from build123d import *

# Parameters (mm, degrees)
SKETCH1_W           = 82.539998569
SKETCH1_H           = 65.04
BOSS_EXTRUDE1_DEPTH = 43.18
SHELL1_T            = 2.54
SKETCH2_R           = 1.085
CUT_EXTRUDE1_DEPTH  = 124.952130409
FILLET1_R           = 6.20014
FILLET2_R           = 1
SKETCH6_W           = 35.56
SKETCH6_H           = 50.8
CUT_EXTRUDE2_DEPTH  = 124.028758627
SKETCH3_R           = 2.125
BOSS_EXTRUDE2_DEPTH = 9.39038
CUT_EXTRUDE3_DEPTH  = 2.54
SKETCH8_W           = 1.27
SKETCH8_H           = 33.02
CUT_EXTRUDE4_DEPTH  = 2.54
SKETCH10_W          = 87.619998569
SKETCH10_H          = 10.145268184
BOSS_EXTRUDE3_DEPTH = 2.54
CUT_EXTRUDE5_DEPTH  = 2.54
SKETCH11_W          = 12.7
SKETCH11_H          = 8
BOSS_EXTRUDE4_DEPTH = 12.7
SKETCH12_R          = 2.625
CUT_EXTRUDE6_DEPTH  = 127.362400741
SKETCH13_W          = 7.62
SKETCH13_H          = 12.7
BOSS_EXTRUDE5_DEPTH = 12.7
SKETCH14_R          = 2.625
CUT_EXTRUDE7_DEPTH  = 125.717897357
FILLET3_R           = 3


with BuildPart() as part:
    # Sketch1 → Boss-Extrude1 (new body)
    with BuildSketch(Plane.XY):
        with Locations((47.599999189, 40.75)):
            Rectangle(SKETCH1_W, SKETCH1_H)
    extrude(amount=BOSS_EXTRUDE1_DEPTH)

    # Shell1
    shell1_openings = [part.faces().sort_by_distance(p)[0] for p in [
        (47.599999189, 73.27, 21.59),
        (47.599999189, 40.75, 0),
    ]]
    offset(amount=SHELL1_T, openings=shell1_openings, kind=Kind.INTERSECTION)

    # Sketch2 → Cut-Extrude1 (cut, through all)
    with BuildSketch(Plane(origin=(97.099998474, 5.69, 0), x_dir=(0, 0, -1), z_dir=(0, 1, 0))):
        with Locations(Location((-10.166, 73.199999285, 0), (0, 0, 90))):
            Circle(SKETCH2_R)
        with Locations(Location((-10.166, 25.799999285, 0), (0, 0, 90))):
            Circle(SKETCH2_R)
        with Locations(Location((-28.266, 24.299999285, 0), (0, 0, 90))):
            Circle(SKETCH2_R)
        with Locations(Location((-28.266, 74.699999285, 0), (0, 0, 90))):
            Circle(SKETCH2_R)
        Polygon((-33.02, 71.391050497), (-8.912, 71.391050497), (-8.912, 55.244166488), (-6.912, 55.244166488), (-6.912, 43.755832082), (-8.912, 43.755832082), (-8.912, 27.608948073), (-33.02, 27.608948073), align=None)
    extrude(amount=CUT_EXTRUDE1_DEPTH, mode=Mode.SUBTRACT)

    # Fillet1
    fillet1_edges = [part.edges().sort_by_distance(p)[0] for p in [
        (25.708947978, 6.96, 33.02),
        (69.491050401, 6.96, 33.02),
        (69.491050401, 6.96, 8.912),
        (25.708947978, 6.96, 8.912),
    ]]
    fillet(fillet1_edges, radius=FILLET1_R)

    # Fillet2
    fillet2_edges = [part.edges().sort_by_distance(p)[0] for p in [
        (53.344166393, 6.96, 6.912),
        (41.855831986, 6.96, 6.912),
    ]]
    fillet(fillet2_edges, radius=FILLET2_R)
    fillet2_2_edges = [part.edges().sort_by_distance(p)[0] for p in [
        (53.344166393, 6.96, 8.912),
        (41.855831986, 6.96, 8.912),
    ]]
    fillet(fillet2_2_edges, radius=FILLET2_R - 0.0001)  # a hair under: the kernel refuses the full size

    # Sketch6 → Cut-Extrude2 (cut, through all)
    with BuildSketch(Plane.ZY.offset(-3.789999905)):
        with Locations((17.78, 47.87)):
            Rectangle(SKETCH6_W, SKETCH6_H)
    extrude(amount=-CUT_EXTRUDE2_DEPTH, mode=Mode.SUBTRACT)

    # Sketch3 → Boss-Extrude2 (add)
    # profile 1 of 4: a face of its own
    with BuildSketch(Plane(origin=(0, 0, 43.18), x_dir=(-1, 0, 0), z_dir=(0, 0, -1))):
        with BuildLine():
            Line((-86.514394884, 72), (-78.685601874, 72))
            ThreePointArc((-78.685601874, 72), (-78.109870373, 62.509871885), (-87.599998474, 63.085603617))
            Line((-87.599998474, 63.085603617), (-87.599998474, 70.914396383))
            ThreePointArc((-87.599998474, 70.914396383), (-87.090126494, 71.490128006), (-86.514394884, 72))
        make_face()
        with Locations(Location((-82.599998379, 67, 0), (0, 0, 180))):
            Circle(SKETCH3_R, mode=Mode.SUBTRACT)
    # profile 2 of 4: a face of its own
    with BuildSketch(Plane(origin=(0, 0, 43.18), x_dir=(-1, 0, 0), z_dir=(0, 0, -1))):
        with BuildLine():
            Line((-7.599999905, 70.914398454), (-7.599999905, 63.085601546))
            ThreePointArc((-7.599999905, 63.085601546), (-17.090127314, 62.509872815), (-16.514394884, 72))
            Line((-16.514394884, 72), (-8.685601874, 72))
            ThreePointArc((-8.685601874, 72), (-8.109871193, 71.490128936), (-7.599999905, 70.914398454))
        make_face()
        with Locations(Location((-12.599998379, 67, 0), (0, 0, 180))):
            Circle(SKETCH3_R, mode=Mode.SUBTRACT)
    # profile 3 of 4: a face of its own
    with BuildSketch(Plane(origin=(0, 0, 43.18), x_dir=(-1, 0, 0), z_dir=(0, 0, -1))):
        with BuildLine():
            Line((-7.599999905, 20.914398454), (-7.599999905, 13.085601546))
            ThreePointArc((-7.599999905, 13.085601546), (-18.949998379, 17), (-7.599999905, 20.914398454))
        make_face()
        with Locations(Location((-12.599998379, 17, 0), (0, 0, 180))):
            Circle(SKETCH3_R, mode=Mode.SUBTRACT)
    # profile 4 of 4: a face of its own
    with BuildSketch(Plane(origin=(0, 0, 43.18), x_dir=(-1, 0, 0), z_dir=(0, 0, -1))):
        with BuildLine():
            Line((-87.599998474, 20.914396383), (-87.599998474, 13.085603617))
            ThreePointArc((-87.599998474, 13.085603617), (-76.249998379, 17), (-87.599998474, 20.914396383))
        make_face()
        with Locations(Location((-82.599998379, 17, 0), (0, 0, 180))):
            Circle(SKETCH3_R, mode=Mode.SUBTRACT)
    extrude(amount=BOSS_EXTRUDE2_DEPTH)

    # Sketch7 → Cut-Extrude3 (cut)
    with BuildSketch(Plane(origin=(0, 0, 0), x_dir=(-1, 0, 0), z_dir=(0, 0, -1))):
        Polygon((-91.409998474, 22.47), (-90.139998474, 22.47), (-90.139998474, 6.96), (-5.059999905, 6.96), (-5.059999905, 22.47), (-3.789999905, 22.47), (-3.789999905, 5.69), (-91.409998474, 5.69), align=None)
    extrude(amount=-CUT_EXTRUDE3_DEPTH, mode=Mode.SUBTRACT)

    # Sketch8 → Cut-Extrude4 (cut)
    with BuildSketch(Plane(origin=(0, 22.47, 0), x_dir=(1, 0, 0), z_dir=(0, 1, 0))):
        with Locations((4.424999905, -19.05)):
            Rectangle(SKETCH8_W, SKETCH8_H)
        with Locations((90.774998474, -19.05)):
            Rectangle(SKETCH8_W, SKETCH8_H)
    extrude(amount=-CUT_EXTRUDE4_DEPTH, mode=Mode.SUBTRACT)

    # Sketch10 → Boss-Extrude3 (add)
    with BuildSketch(Plane(origin=(0, 73.27, 0), x_dir=(1, 0, 0), z_dir=(0, 1, 0))):
        with Locations((47.59999919, -40.647365908)):
            Rectangle(SKETCH10_W, SKETCH10_H)
    extrude(amount=BOSS_EXTRUDE3_DEPTH)

    # Sketch9 → Cut-Extrude5 (cut)
    with BuildSketch(Plane(origin=(0, 0, 35.56), x_dir=(-1, 0, 0), z_dir=(0, 0, -1))):
        Polygon((-90.139998474, 73.27), (-90.139998474, 74.54), (-5.059999905, 74.54), (-5.059999905, 73.27), (-5.059999905, 19.93), (-3.789999905, 19.93), (-3.789999905, 73.27), (-3.789999905, 75.81), (-91.409998474, 75.81), (-91.409998474, 73.27), (-91.409998474, 19.93), (-90.139998474, 19.93), align=None)
    extrude(amount=-CUT_EXTRUDE5_DEPTH, mode=Mode.SUBTRACT)

    # Sketch11 → Boss-Extrude4 (add)
    with BuildSketch(Plane.XZ.offset(-5.69)):
        with Locations((83.789998474, 6.54)):
            Rectangle(SKETCH11_W, SKETCH11_H)
        with Locations((11.409999905, 6.54)):
            Rectangle(SKETCH11_W, SKETCH11_H)
    extrude(amount=BOSS_EXTRUDE4_DEPTH)

    # Sketch12 → Cut-Extrude6 (cut, through all)
    with BuildSketch(Plane(origin=(0, 0, 2.54), x_dir=(-1, 0, 0), z_dir=(0, 0, -1))):
        with Locations((-83.789998474, -0.66)):
            Circle(SKETCH12_R)
        with Locations((-11.409999905, -0.66)):
            Circle(SKETCH12_R)
    extrude(amount=-CUT_EXTRUDE6_DEPTH, mode=Mode.SUBTRACT)

    # Sketch13 → Boss-Extrude5 (add)
    with BuildSketch(Plane.ZY.offset(-3.789999905)):
        with Locations((41.91, 69.46)):
            Rectangle(SKETCH13_W, SKETCH13_H)
    boss_extrude5 = extrude(amount=BOSS_EXTRUDE5_DEPTH)

    # Sketch14 → Cut-Extrude7 (cut, through all)
    with BuildSketch(Plane(origin=(0, 0, 38.1), x_dir=(-1, 0, 0), z_dir=(0, 0, -1))):
        with Locations(Location((2.560000095, 69.46, 0), (0, 0, 90))):
            Circle(SKETCH14_R)
    cut_extrude7 = extrude(amount=-CUT_EXTRUDE7_DEPTH, mode=Mode.SUBTRACT)

    # Mirror1: Boss-Extrude5, Cut-Extrude7 across plane
    add(boss_extrude5.mirror(Plane.ZY.offset(-47.599999189)))
    add(cut_extrude7.mirror(Plane.ZY.offset(-47.599999189)), mode=Mode.SUBTRACT)

    # Fillet3
    fillet3_edges = [part.edges().sort_by_distance(p)[0] for p in [
        (6.329999905, 73.27, 39.377365908),
        (6.329999905, 8.23, 21.59),
        (88.869998474, 8.23, 21.59),
        (88.869998474, 73.27, 39.377365908),
        (17.759999905, 5.69, 6.54),
        (17.759999905, -7.01, 6.54),
        (5.059999905, -7.01, 6.54),
        (77.439998474, 5.69, 6.54),
        (90.139998474, -7.01, 6.54),
        (77.439998474, -7.01, 6.54),
        (3.789999905, 63.11, 41.91),
        (-8.910000095, 63.11, 41.91),
        (-8.910000095, 75.81, 41.91),
        (104.109998474, 75.81, 41.91),
        (104.109998474, 63.11, 41.91),
        (91.409998474, 63.11, 41.91),
        (91.409998474, 5.69, 24.13),
        (3.789999905, 5.69, 24.13),
    ]]
    fillet(fillet3_edges, radius=FILLET3_R)


solid = part.part
Here's how the part is built. I have some questions about the finished solid (model axes, mm). A direction names the side the tool comes from. Give positions to 0.01 mm unless a question says otherwise; leave off trailing zeros. Order: outer loops, then holes, each group sorted by start corner. A loop starts at its lowest first (then second) coordinate and runs counter-clockwise, first axis right, second up. Notation, with made-up numbers: (56, -2.5) -> (91, -2.5) arc R20 cw to (91, 1.5) -> close; hole circle Ø3 at (33.25, 0.25). An arc over 180 degrees is marked (long way). Use a Markdown table: item, result. Add a question column.
Item 1: Imagine slicing it at D-D on y = 45.5. Please give me the cut outline in (x, z), plus the area to 3 significant figures.
Item 2: Imagine slicing it at C-C on z = 20. Please give me the cut outline in (x, y), plus the area to 3 significant figures.
Item 3: For faces 1 (the face through (7.23, 9.09, 21.89)), 2 (the face through (67.63, 6.98, 31.25)), 3 (the face through (98, 63.11, 42)), which set-ups out of +Z, -Z, +X, -X, +Y, -Y let a thin tool reach every point of the face, with its end or its side?
Item 4: Imagine slicing it at A-A on x = -2.56. Please give me the cut outline in (y, z) (3 decimals).
Item 5: If we mould it in two halves opening along X, with no side actions, what happens to faces 4 (the face through (8.906, 0.128, 6.484)), 5 (the face through (103.21, 63.97, 41.96)), 6 (the face through (78.3, -6.11, 6.6)), 7 (the face through (-8.01, 74.95, 41.96))? For each: pulls with the +X half, pulls with the -X half, needs draft (parallel to the pull), parting line crosses it, or undercut.
Item 6: I need wall thicknesses on line 1 (X direction, y = -1, z = 3); line 2 (Z direction, x = 72.8, y = 7.3); line 3 (X direction, y = 12.5, z = 31.5). Which ranges of each line are inside material? Lowest first, please.
Item 7: Will these pins go through, and if not, where does the flat tip stop? pin 1 (5 mm diameter, centred on x = 71, y = 43.5, fed in from -Z); pin 2 (12.5 mm diameter, centred on x = 13.5, y = 19, fed in from -Z); pin 3 (2 mm diameter, centred on y = 7, z = 21.5, fed in from +X); pin 4 (13 mm diameter, centred on x = 34, z = 16, fed in from +Y).
Item 8: Imagine slicing it at B-B on y = -0.66. Please give me the cut outline in (x, z) (3 decimals), plus the area to 3 significant figures.
Data:
| question | item | result |
|---|---|---|
| 1 | outline | (3.79, 38.1) -> (5.06, 38.1) -> (5.06, 35.56) -> (6.33, 35.56) -> (6.33, 43.18) -> (88.87, 43.18) -> (88.87, 35.56) -> (90.14, 35.56) -> (90.14, 38.1) -> (91.41, 38.1) -> (91.41, 45.72) -> (3.79, 45.72) -> close |
| 1 | area | 255 mm² |
| 2 | outline | (3.79, 8.69) arc R3 ccw to (6.79, 5.69) -> (25.71, 5.69) -> (25.71, 8.23) -> (9.33, 8.23) arc R3 cw to (6.33, 11.23) -> (6.33, 22.47) -> (5.06, 22.47) -> (5.06, 19.93) -> (3.79, 19.93) -> close; (69.49, 5.69) -> (88.41, 5.69) arc R3 ccw to (91.41, 8.69) -> (91.41, 19.93) -> (90.14, 19.93) -> (90.14, 22.47) -> (88.87, 22.47) -> (88.87, 11.23) arc R3 cw to (85.87, 8.23) -> (69.49, 8.23) -> close |
| 2 | area | 177 mm² |
| 3 | face 1 | -Z |
| 3 | face 2 | +Y, -Y |
| 3 | face 3 | +Z, -Z, +X, -Y |
| 4 | outline | (63.11, 38.1) -> (66.835, 38.1) -> (66.835, 45.72) -> (63.11, 45.72) -> close; (72.085, 38.1) -> (75.81, 38.1) -> (75.81, 45.72) -> (72.085, 45.72) -> close |
| 5 | face 4 | undercut |
| 5 | face 5 | pulls with the +X half |
| 5 | face 6 | undercut |
| 5 | face 7 | pulls with the -X half |
| 6 | line 1 | x = 5.06 to 8.81, 14.01 to 17.76, 77.44 to 81.19, 86.39 to 90.14 |
| 6 | line 2 | z = 0 to 27.18, 29.35 to 45.72 |
| 6 | line 3 | x = 3.79 to 6.33, 88.87 to 91.41 |
| 7 | pin 1 | stops at z = 43.18 |
| 7 | pin 2 | stops at z = 33.79 |
| 7 | pin 3 | stops at x = 91.33 |
| 7 | pin 4 | passes through |
| 8 | outline | (5.06, 2.54) -> (8.785, 2.54) -> (8.785, 10.54) -> (5.06, 10.54) -> close; (14.035, 2.54) -> (17.76, 2.54) -> (17.76, 10.54) -> (14.035, 10.54) -> close; (77.44, 2.54) -> (81.165, 2.54) -> (81.165, 10.54) -> (77.44, 10.54) -> close; (86.415, 2.54) -> (90.14, 2.54) -> (90.14, 10.54) -> (86.415, 10.54) -> close |
| 8 | area | 119 mm² |
